from build123d import *

# Parameters (mm, degrees)
SKETCH_W        = 37
SKETCH_H        = 40
PAD_DEPTH       = 10
SKETCH001_W     = 33
SKETCH001_H     = 33
POCKET_DEPTH    = 9
POCKET001_DEPTH = 40.001
SKETCH003_R     = 0.75
SKETCH003_R_2   = 0.4
POCKET002_DEPTH = 10.001


with BuildPart() as part:
    # Sketch → Pad (new body)
    with BuildSketch(Plane.XY):
        Rectangle(SKETCH_W, SKETCH_H)
    extrude(amount=PAD_DEPTH)

    # Sketch001 (on Face6 of Pad) → Pocket (cut)
    with BuildSketch(Plane.XY.offset(10)):
        Rectangle(SKETCH001_W, SKETCH001_H)
    extrude(amount=-POCKET_DEPTH, mode=Mode.SUBTRACT)

    # Sketch002 (on Face1 of Pocket) → Pocket001 (cut, through all)
    with BuildSketch(Plane(origin=(0, 20, 0), x_dir=(-1, 0, 0), z_dir=(0, 1, 0))):
        Polygon((14.424978, 20.424978), (0, 6), (-14.424978, 20.424978), align=None)
    extrude(amount=-POCKET001_DEPTH, mode=Mode.SUBTRACT)

    # Sketch003 (on Face7 of Pocket001) → Pocket002 (cut, through all)
    with BuildSketch(Plane.XY.offset(10)):
        with Locations((-10, 18)):
            Circle(SKETCH003_R)
        with Locations((10, 18)):
            Circle(SKETCH003_R_2)
        with Locations((-10, -18)):
            Circle(SKETCH003_R_2)
        with Locations((10, -18)):
            Circle(SKETCH003_R)
    extrude(amount=-POCKET002_DEPTH, mode=Mode.SUBTRACT)


solid = part.part
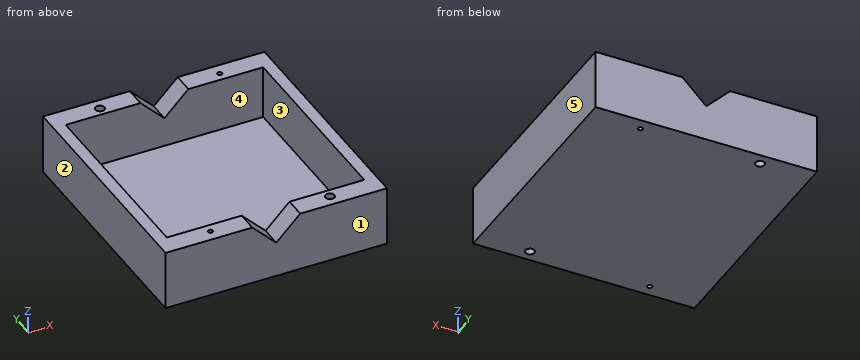
Input: part model. Units: mm. Frame: model coordinates. Face numbers are marked on the shaded views. A direction names the side the tool comes from. Give positions to 0.01 mm unless a question says otherwise; leave off trailing zeros. Order: outer loops, then holes, each group sorted by start corner. A loop starts at its lowest first (then second) coordinate and runs counter-clockwise, first axis right, second up. Notation, with made-up numbers: M 79,-14.5 L 111,-14.5 A28 cw 111,14.5 Z; hole C 58.5,20.25 d4. An arc over 180 degrees is marked long. Answer as a JSON object with one key per item and string values.
1. Cut plane C-C, the plane x = 7.5. Output: boundary loops of the cut face in (y, z), and give its area (3 significant figures).
Result sheet:
{"outline": "M -20,0 L 20,0 L 20,10 L 16.5,10 L 16.5,1 L -16.5,1 L -16.5,10 L -20,10 Z", "area": "103 mm²"}
2. Cut plane A-A, the plane z = 7. Output: boundary loops of the cut face in (x, y), and give its area (3 significant figures).
Result sheet:
{"outline": "M -18.5,-20 L -1,-20 L -1,-16.5 L -16.5,-16.5 L -16.5,16.5 L -1,16.5 L -1,20 L -18.5,20 Z; M 1,-20 L 18.5,-20 L 18.5,20 L 1,20 L 1,16.5 L 16.5,16.5 L 16.5,-16.5 L 1,-16.5 Z; hole C -10,18 d1.5; hole C -10,-18 d0.8; hole C 10,-18 d1.5; hole C 10,18 d0.8", "area": "372 mm²"}
3. Cut plane B-B, the plane z = 2.5. Output: boundary loops of the cut face in (x, y).
Result sheet:
{"outline": "M -18.5,-20 L 18.5,-20 L 18.5,20 L -18.5,20 Z; hole M -16.5,-16.5 L 16.5,-16.5 L 16.5,16.5 L -16.5,16.5 Z; hole C -10,18 d1.5; hole C -10,-18 d0.8; hole C 10,-18 d1.5; hole C 10,18 d0.8"}
4. Reachability of the marked faces 4 and 5 from +Z, -Z, +X, -X, +Y, -Y: full face, straight path, thin tool, end or side. Return the list, or none.
Result sheet:
{"face 4": "+Z", "face 5": "+Z, -Z, +X, +Y, -Y"}
5. Pull-direction query (Y, two-part tool) for the marked faces 1, 2 and 3; classes: +Y half, -Y half, draft (parallel to the pull), parting line (faces both ways), or undercut.
Result sheet:
{"face 1": "-Y half", "face 2": "draft", "face 3": "undercut"}
6. First-contact query: P1, Ø2.5, axis at x = -10, y = 18, coming from the +Z side; P2, Ø10, axis at x = 0, y = 5, coming from the +Z side. Flat tips, straight axial feed; report the tip coordinate or a pass-through.
Result sheet:
{"P1": "z = 10", "P2": "z = 1"}
7. Cut plane D-D, the plane y = -2. Output: boundary loops of the cut face in (x, z).
Result sheet:
{"outline": "M -18.5,0 L 18.5,0 L 18.5,10 L 16.5,10 L 16.5,1 L -16.5,1 L -16.5,10 L -18.5,10 Z"}
8. Ray query, line 1 (Y direction, x = 10, z = 5.25); line 2 (Y direction, x = -10, z = 6.75); line 3 (Y direction, x = -14, z = 4.75). Return the intervals inside material, ascending. Write a range as [from, to].
Result sheet:
{"line 1": "[-20, -18.75], [-17.25, -16.5], [16.5, 17.6], [18.4, 20]", "line 2": "[-20, -18.4], [-17.6, -16.5], [16.5, 17.25], [18.75, 20]", "line 3": "[-20, -16.5], [16.5, 20]"}
